Source: three-view drawing plus pictorial views. Frame: mm from the lowest corner of the part. A direction names the side the tool comes from. Round coordinates to 2 decimals unless told otherwise and drop trailing zeros. Write each loop counter-clockwise with the first axis right and the second up, starting at its lowest first coordinate (ties: lowest second). Pieces come first, ordered by that corner, then holes. Notation, with made-up numbers: (-28, 78) - (16, 78) arc R22 cw to (16, 108) - close; hole circle Ø4 at (38.25, -9.75). An arc over 180 degrees is marked (long way). Write each question's results on one line, items separated by ' | '.
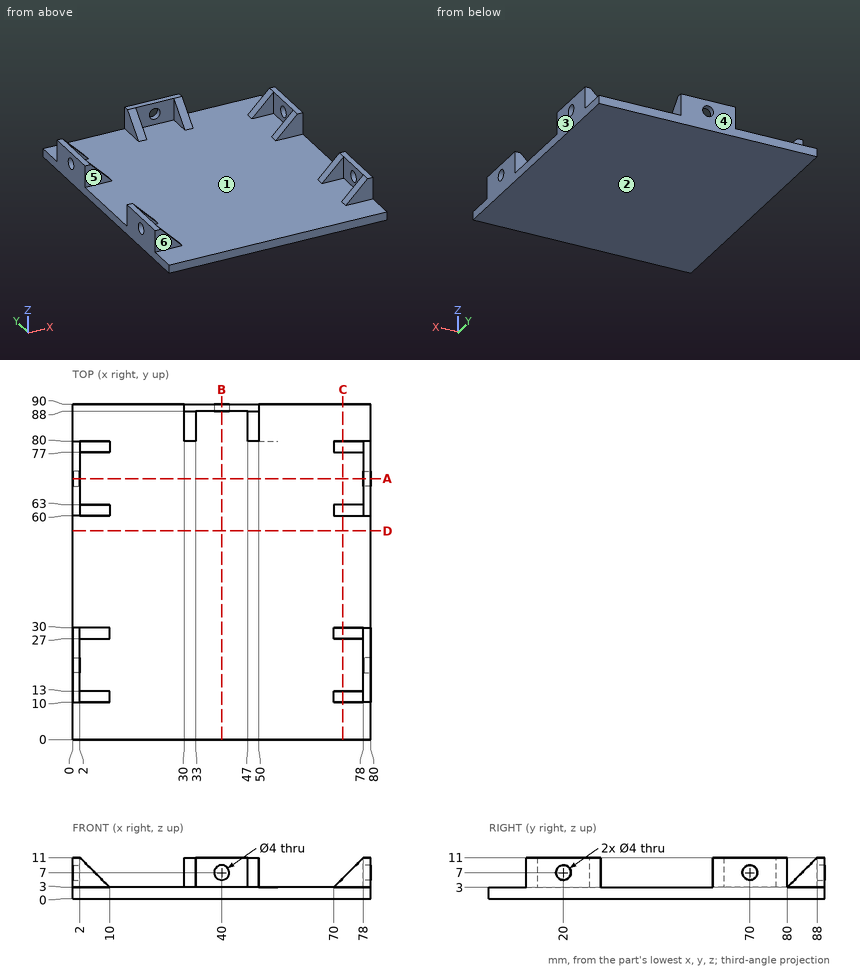
Q1. Pin query (flat end, axial travel): pin 1 (4 mm diameter, centred on x = 5, z = 6, fed in from +Y); pin 2 (2.5 mm diameter, centred on x = 6.5, z = 7, fed in from -Y); pin 3 (12 mm diameter, centred on x = 33, y = 17, fed in from +Z); pin 4 (3.5 mm diameter, centred on y = 20, z = 7, fed in from -X). Return the tip coordinate at first contact, or that it passes through.
Answer block:
pin 1: y = 80 | pin 2: y = 10 | pin 3: z = 3 | pin 4: through
Q2. Section query D-D, the plane y = 56. Return loops of the section in (x, z).
Answer block:
outline: (0, 0) - (80, 0) - (80, 3) - (0, 3) - close
Q3. Section query A-A, the plane y = 70. Return loops of the section in (x, z).
Answer block:
outline: (0, 0) - (80, 0) - (80, 5) - (78, 5) - (78, 3) - (2, 3) - (2, 5) - (0, 5) - close; (0, 9) - (2, 9) - (2, 11) - (0, 11) - close; (78, 9) - (80, 9) - (80, 11) - (78, 11) - close
Q4. Access query for the marked faces 1 and 2. Directions: +Z, -Z, +X, -X, +Y, -Y. A direction counts if a zero-diameter tool reaches every point of the face in a straight line with its end or side. Return the directions, or none.
Answer block:
face 1: +Z | face 2: -Z, +X, -X, +Y, -Y
Q5. Section query B-B, the plane x = 40. Return loops of the section in (y, z).
Answer block:
outline: (0, 0) - (90, 0) - (90, 5) - (88, 5) - (88, 3) - (0, 3) - close; (88, 9) - (90, 9) - (90, 11) - (88, 11) - close
Q6. Mould query, pull axis Y, two halves, no side actions, for the marked faces 3, 4, 5 and 6. Classes: pulls with the +Y half, pulls with the -Y half, needs draft (parallel to the pull), parting line crosses it, or undercut.
Answer block:
face 3: needs draft | face 4: pulls with the +Y half | face 5: undercut | face 6: pulls with the -Y half
Q7. Section query C-C, the plane x = 72.5. Return loops of the section in (y, z).
Answer block:
outline: (0, 0) - (90, 0) - (90, 3) - (80, 3) - (80, 5.5) - (77, 5.5) - (77, 3) - (63, 3) - (63, 5.5) - (60, 5.5) - (60, 3) - (30, 3) - (30, 5.5) - (27, 5.5) - (27, 3) - (13, 3) - (13, 5.5) - (10, 5.5) - (10, 3) - (0, 3) - close
Q8. Ray query, line 1 along X through (y, z) = (88.8, 7); line 2 along X through (y, z) = (23, 7); line 3 along Y through (x, z) = (34, 9). Return the intervals inside material, ascending.
Answer block:
line 1: 30 to 38, 42 to 50 | line 2: 0 to 2, 78 to 80 | line 3: 88 to 90
